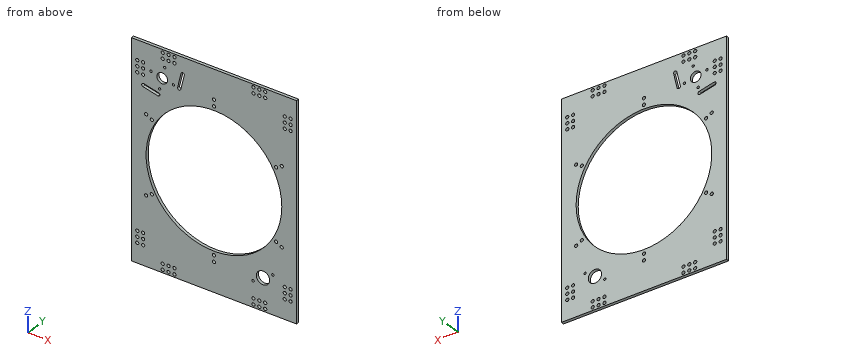
```python
from build123d import *

# Parameters (mm, degrees)
SKETCH1_W           = 355.6
SKETCH1_H           = 463.55
SKETCH1_R           = 146.05
SKETCH1_R_2         = 3.429
SKETCH1_R_3         = 2.54
SKETCH1_R_4         = 11.43
SKETCH1_R_5         = 14.2875
BOSS_EXTRUDE1_DEPTH = 6.35


with BuildPart() as part:
    # Sketch1 → Boss-Extrude1 (new body)
    with BuildSketch(Plane(origin=(0, 0, 0), x_dir=(1, 0, 0), z_dir=(0, 1, 0))):
        Rectangle(SKETCH1_W, SKETCH1_H)
        Circle(SKETCH1_R, mode=Mode.SUBTRACT)
        with Locations((0, 168.5)):
            Circle(SKETCH1_R_2, mode=Mode.SUBTRACT)
        with Locations((145.925280538, 84.25)):
            Circle(SKETCH1_R_2, mode=Mode.SUBTRACT)
        with Locations((145.925280538, -84.25)):
            Circle(SKETCH1_R_2, mode=Mode.SUBTRACT)
        with Locations((0, -168.5)):
            Circle(SKETCH1_R_2, mode=Mode.SUBTRACT)
        with Locations((-145.925280538, -84.25)):
            Circle(SKETCH1_R_2, mode=Mode.SUBTRACT)
        with Locations((-145.925280538, 84.25)):
            Circle(SKETCH1_R_2, mode=Mode.SUBTRACT)
        with Locations((-165.1, 189.7126)):
            Circle(SKETCH1_R_2, mode=Mode.SUBTRACT)
        with Locations((-152.4, 189.7126)):
            Circle(SKETCH1_R_2, mode=Mode.SUBTRACT)
        with Locations((-152.4, 177.0126)):
            Circle(SKETCH1_R_2, mode=Mode.SUBTRACT)
        with Locations((-165.1, 177.0126)):
            Circle(SKETCH1_R_2, mode=Mode.SUBTRACT)
        with Locations((-152.4, 164.3126)):
            Circle(SKETCH1_R_2, mode=Mode.SUBTRACT)
        with Locations((-165.1, 164.3126)):
            Circle(SKETCH1_R_2, mode=Mode.SUBTRACT)
        with Locations((165.1, 164.3126)):
            Circle(SKETCH1_R_2, mode=Mode.SUBTRACT)
        with Locations((152.4, 164.3126)):
            Circle(SKETCH1_R_2, mode=Mode.SUBTRACT)
        with Locations((165.1, 177.0126)):
            Circle(SKETCH1_R_2, mode=Mode.SUBTRACT)
        with Locations((152.4, 177.0126)):
            Circle(SKETCH1_R_2, mode=Mode.SUBTRACT)
        with Locations((152.4, 189.7126)):
            Circle(SKETCH1_R_2, mode=Mode.SUBTRACT)
        with Locations((165.1, 189.7126)):
            Circle(SKETCH1_R_2, mode=Mode.SUBTRACT)
        with Locations((165.1, -189.7126)):
            Circle(SKETCH1_R_2, mode=Mode.SUBTRACT)
        with Locations((152.4, -189.7126)):
            Circle(SKETCH1_R_2, mode=Mode.SUBTRACT)
        with Locations((152.4, -177.0126)):
            Circle(SKETCH1_R_2, mode=Mode.SUBTRACT)
        with Locations((165.1, -177.0126)):
            Circle(SKETCH1_R_2, mode=Mode.SUBTRACT)
        with Locations((152.4, -164.3126)):
            Circle(SKETCH1_R_2, mode=Mode.SUBTRACT)
        with Locations((165.1, -164.3126)):
            Circle(SKETCH1_R_2, mode=Mode.SUBTRACT)
        with Locations((-165.1, -164.3126)):
            Circle(SKETCH1_R_2, mode=Mode.SUBTRACT)
        with Locations((-152.4, -164.3126)):
            Circle(SKETCH1_R_2, mode=Mode.SUBTRACT)
        with Locations((-165.1, -177.0126)):
            Circle(SKETCH1_R_2, mode=Mode.SUBTRACT)
        with Locations((-152.4, -177.0126)):
            Circle(SKETCH1_R_2, mode=Mode.SUBTRACT)
        with Locations((-152.4, -189.7126)):
            Circle(SKETCH1_R_2, mode=Mode.SUBTRACT)
        with Locations((-165.1, -189.7126)):
            Circle(SKETCH1_R_2, mode=Mode.SUBTRACT)
        with Locations((-110.3376, 225.425)):
            Circle(SKETCH1_R_2, mode=Mode.SUBTRACT)
        with Locations((-97.6376, 225.425)):
            Circle(SKETCH1_R_2, mode=Mode.SUBTRACT)
        with Locations((-84.9376, 225.425)):
            Circle(SKETCH1_R_2, mode=Mode.SUBTRACT)
        with Locations((-97.6376, 212.725)):
            Circle(SKETCH1_R_2, mode=Mode.SUBTRACT)
        with Locations((-84.9376, 212.725)):
            Circle(SKETCH1_R_2, mode=Mode.SUBTRACT)
        with Locations((-110.3376, 212.725)):
            Circle(SKETCH1_R_2, mode=Mode.SUBTRACT)
        with Locations((110.3376, 212.725)):
            Circle(SKETCH1_R_2, mode=Mode.SUBTRACT)
        with Locations((84.9376, 212.725)):
            Circle(SKETCH1_R_2, mode=Mode.SUBTRACT)
        with Locations((97.6376, 212.725)):
            Circle(SKETCH1_R_2, mode=Mode.SUBTRACT)
        with Locations((84.9376, 225.425)):
            Circle(SKETCH1_R_2, mode=Mode.SUBTRACT)
        with Locations((97.6376, 225.425)):
            Circle(SKETCH1_R_2, mode=Mode.SUBTRACT)
        with Locations((110.3376, 225.425)):
            Circle(SKETCH1_R_2, mode=Mode.SUBTRACT)
        with Locations((110.3376, -225.425)):
            Circle(SKETCH1_R_2, mode=Mode.SUBTRACT)
        with Locations((97.6376, -225.425)):
            Circle(SKETCH1_R_2, mode=Mode.SUBTRACT)
        with Locations((84.9376, -225.425)):
            Circle(SKETCH1_R_2, mode=Mode.SUBTRACT)
        with Locations((97.6376, -212.725)):
            Circle(SKETCH1_R_2, mode=Mode.SUBTRACT)
        with Locations((84.9376, -212.725)):
            Circle(SKETCH1_R_2, mode=Mode.SUBTRACT)
        with Locations((110.3376, -212.725)):
            Circle(SKETCH1_R_2, mode=Mode.SUBTRACT)
        with Locations((-110.3376, -212.725)):
            Circle(SKETCH1_R_2, mode=Mode.SUBTRACT)
        with Locations((-84.9376, -212.725)):
            Circle(SKETCH1_R_2, mode=Mode.SUBTRACT)
        with Locations((-97.6376, -212.725)):
            Circle(SKETCH1_R_2, mode=Mode.SUBTRACT)
        with Locations((-84.9376, -225.425)):
            Circle(SKETCH1_R_2, mode=Mode.SUBTRACT)
        with Locations((-97.6376, -225.425)):
            Circle(SKETCH1_R_2, mode=Mode.SUBTRACT)
        with Locations((-110.3376, -225.425)):
            Circle(SKETCH1_R_2, mode=Mode.SUBTRACT)
        with Locations((-116.969340251, -147.611717522)):
            Circle(SKETCH1_R_3, mode=Mode.SUBTRACT)
        with Locations((-87.146214855, -166.979081607)):
            Circle(SKETCH1_R_3, mode=Mode.SUBTRACT)
        with Locations((-105.904201711, -195.863848358)):
            Circle(SKETCH1_R_3, mode=Mode.SUBTRACT)
        with Locations((-135.562836399, -177.27035221)):
            Circle(SKETCH1_R_3, mode=Mode.SUBTRACT)
        with Locations((-111.436770981, -171.73778294)):
            Circle(SKETCH1_R_4, mode=Mode.SUBTRACT)
        with Locations((105.605508889, 162.618223125)):
            Circle(SKETCH1_R_5, mode=Mode.SUBTRACT)
        with Locations((84.303276464, 176.452054614)):
            Circle(SKETCH1_R_3, mode=Mode.SUBTRACT)
        with Locations((126.907741315, 148.784391635)):
            Circle(SKETCH1_R_3, mode=Mode.SUBTRACT)
        with Locations((0, 154.5)):
            Circle(SKETCH1_R_2, mode=Mode.SUBTRACT)
        with Locations((133.800924885, 77.25)):
            Circle(SKETCH1_R_2, mode=Mode.SUBTRACT)
        with Locations((133.800924885, -77.25)):
            Circle(SKETCH1_R_2, mode=Mode.SUBTRACT)
        with Locations((0, -154.5)):
            Circle(SKETCH1_R_2, mode=Mode.SUBTRACT)
        with Locations((-133.800924885, -77.25)):
            Circle(SKETCH1_R_2, mode=Mode.SUBTRACT)
        with Locations((-133.800924885, 77.25)):
            Circle(SKETCH1_R_2, mode=Mode.SUBTRACT)
        with BuildLine():
            Line((-71.301492569, -163.345583061), (-63.920948648, -195.530175204))
            ThreePointArc((-63.920948648, -195.530175204), (-66.592153841, -199.791036011), (-70.853014648, -197.119830818))
            Line((-70.853014648, -197.119830818), (-78.233558569, -164.935238675))
            ThreePointArc((-78.233558569, -164.935238675), (-75.562353376, -160.674377868), (-71.301492569, -163.345583061))
        make_face(mode=Mode.SUBTRACT)
        with BuildLine():
            Line((-119.013183183, -138.699061236), (-151.197775326, -146.079605157))
            ThreePointArc((-151.197775326, -146.079605157), (-155.458636133, -143.408399964), (-152.78743094, -139.147539157))
            Line((-152.78743094, -139.147539157), (-120.602838797, -131.766995236))
            ThreePointArc((-120.602838797, -131.766995236), (-116.34197799, -134.438200429), (-119.013183183, -138.699061236))
        make_face(mode=Mode.SUBTRACT)
    extrude(amount=BOSS_EXTRUDE1_DEPTH)


solid = part.part
```
The model under review builds one solid part; all positions refer to its coordinate system, in mm. Coordinates: 2 decimals unless noted, no trailing zeros. Write each loop counter-clockwise with the first axis right and the second up, starting at its lowest first coordinate (ties: lowest second). Pieces come first, ordered by that corner, then holes.
1) We need section A-A on z = 0. State the section outline as (x, y) points, then the cut area to 3 significant figures.
2) We need section C-C on y = 1.25. Count the separate pieces of the cut face and the enclosed holes in it, then the cut area to 3 significant figures.
3) To check wall thickness, follow probe 1 along Z at (x, y) = (0, 1.5) (3 decimals); probe 2 along X at (y, z) = (2.75, -178); probe 3 along Z at (x, y) = (-31.5, 2.25) (3 decimals). State the ranges of each line that lie inside material, in increasing order.
4) We need section B-B on x = -48.5. State the section outline as (y, z) points (3 decimals).
Answer list:
1. outline: (-177.8, 0) - (-146.05, 0) - (-146.05, 6.35) - (-177.8, 6.35) - close; (146.05, 0) - (177.8, 0) - (177.8, 6.35) - (146.05, 6.35) - close
1. area: 403 mm2
2. separate pieces: 1
2. enclosed holes: 71
2. area: 93,900 mm2
3. probe 1: z = -231.775 to -171.929, -165.071 to -157.929, -151.071 to -146.05, 146.05 to 151.071, 157.929 to 165.071, 171.929 to 231.775
3. probe 2: x = -177.8 to -168.38, -161.82 to -155.68, -149.12 to 82.29, 86.32 to 149.12, 155.68 to 161.82, 168.38 to 177.8
3. probe 3: z = -231.775 to -142.613, 142.613 to 231.775
4. outline: (0, -231.775) - (6.35, -231.775) - (6.35, -137.762) - (0, -137.762) - close; (0, 137.762) - (6.35, 137.762) - (6.35, 231.775) - (0, 231.775) - close
